The listing builds one solid part. Answer for the finished solid, in the listing's coordinates (mm). A direction names the side the tool comes from. Give positions to 0.01 mm unless a question says otherwise; leave off trailing zeros. Loops run counter-clockwise (first coordinate to the right, second up) from the corner with the lowest first, then second, coordinate; pieces in that order, holes last. Notation, with made-up numbers: M 83.25,66.25 L 129.25,66.25 A20 ccw 129.25,88.25 Z; hole C -35,50 d4. An arc over 180 degrees is marked long. Return JSON: item names as keys, results as strings.
from build123d import *

# Parameters (mm, degrees)
F0_W     = 130
F0_H     = 70
F1_DEPTH = 50
F2_T     = -2.5
F3_R     = 2.5
F4_DEPTH = 70.001


with BuildPart() as f1:
    # F0 (on Top) → F1 (new body)
    with BuildSketch(Plane.XY):
        Rectangle(F0_W, F0_H)
    extrude(amount=F1_DEPTH)

    # F2
    f2_openings = [f1.faces().sort_by_distance(p)[0] for p in [
        (0, 0, 50),
    ]]
    offset(amount=F2_T, openings=f2_openings)

    # F3 (on face) → F4 (cut, through all)
    with BuildSketch(Plane.XZ.offset(35)):
        with Locations((-56.5, 45)):
            Circle(F3_R)
        with Locations((-44, 45)):
            Circle(F3_R)
        with Locations((-31.5, 45)):
            Circle(F3_R)
        with Locations((-19, 45)):
            Circle(F3_R)
        with Locations((-6.5, 45)):
            Circle(F3_R)
        with Locations((6, 45)):
            Circle(F3_R)
        with Locations((18.5, 45)):
            Circle(F3_R)
        with Locations((31, 45)):
            Circle(F3_R)
        with Locations((43.5, 45)):
            Circle(F3_R)
        with Locations((56, 45)):
            Circle(F3_R)
    extrude(amount=-F4_DEPTH, mode=Mode.SUBTRACT)


solid = f1.part
(1) The part is cut by section C-C (x = -1). Determine the outline of the cut face in (y, z), and give its area (4 significant figures).
Values follow:
{"outline": "M -35,0 L 35,0 L 35,50 L 32.5,50 L 32.5,2.5 L -32.5,2.5 L -32.5,50 L -35,50 Z", "area": "412.5 mm²"}
(2) A tool of negligible diameter and unlimited length cuts with its end or side. For faces 1 (the flat face through (-62.5, 0, 26)), 2 (the cylindrical face through (-21, -33.8, 43.5)), from which of +Z, -Z, +X, -X, +Y, -Y can it reach the whole face along a straight path? Write none if from no direction.
Values follow:
{"face 1": "+Z", "face 2": "+Y, -Y"}
(3) Determine the mould class of faces 3 (the cylindrical face through (5.46, -33.77, 42.56)), 4 (the flat face through (65, 0, 25)), 5 (the flat face through (-1, 0, 2.5)) for opening direction Z: released by +Z, released by -Z, zero draft, split by the parting line, or undercut.
Values follow:
{"face 3": "undercut", "face 4": "zero draft", "face 5": "released by +Z"}
(4) Given pin 1 (4.5 mm diameter, centred on x = 31, z = 45, fed in from -Y); pin 2 (8 mm diameter, centred on x = -37.5, y = 13.5, fed in from +Z), each flat-ended and moving along its own axis, determine where each tip first touches the part or whether it passes through.
Values follow:
{"pin 1": "through", "pin 2": "z = 2.5"}
(5) The part is cut by section B-B (z = 34.5). Determine the outline of the cut face in (x, y), and give its area (3 significant figures).
Values follow:
{"outline": "M -65,-35 L 65,-35 L 65,35 L -65,35 Z; hole M -62.5,-32.5 L 62.5,-32.5 L 62.5,32.5 L -62.5,32.5 Z", "area": "975 mm²"}
(6) Straight lines are drawn through the part: line 1 along Z through (x, y) = (-19, -34); line 2 along Y through (x, z) = (5.5, 3); line 3 along X through (y, z) = (19.5, 42). For each, find the intervals that lie inside material, in ascending order.
Values follow:
{"line 1": "0 to 42.5, 47.5 to 50", "line 2": "-35 to -32.5, 32.5 to 35", "line 3": "-65 to -62.5, 62.5 to 65"}
(7) The part is cut by section A-A (x = -56.5). Determine the outline of the cut face in (y, z), and give its area (4 significant figures).
Values follow:
{"outline": "M -35,0 L 35,0 L 35,42.5 L 32.5,42.5 L 32.5,2.5 L -32.5,2.5 L -32.5,42.5 L -35,42.5 Z; M -35,47.5 L -32.5,47.5 L -32.5,50 L -35,50 Z; M 32.5,47.5 L 35,47.5 L 35,50 L 32.5,50 Z", "area": "387.5 mm²"}
(8) The part is cut by section D-D (y = -28). Determine the outline of the cut face in (x, z).
Values follow:
{"outline": "M -65,0 L 65,0 L 65,50 L 62.5,50 L 62.5,2.5 L -62.5,2.5 L -62.5,50 L -65,50 Z"}
